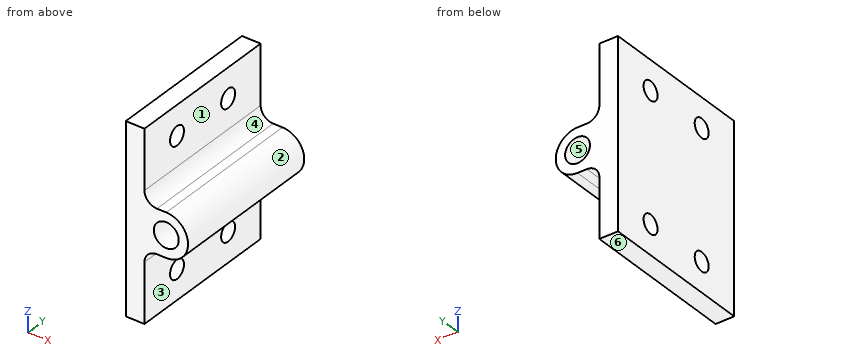
Autodesk Inventor part; units mm, degrees
ref_plane "YZ Plane" through (0, 0, 0) normal (1, 0, 0) x (0, 1, 0)
ref_plane "XZ Plane" through (0, 0, 0) normal (0, 1, 0) x (-1, 0, 0)
ref_plane "XY Plane" through (0, 0, 0) normal (0, 0, 1) x (1, 0, 0)
sketch "Sketch1" plane through (0, 0, 0) normal (0, 1, 0) x (-1, 0, 0)
  line L0 (1.5, 15) -> (-1.5, 15)
  line L1 (-1.5, -15) -> (1.5, -15)
  line L2 (1.5, -15) -> (1.5, 15)
  line L3 (1.5, 15) -> (-1.5, -15) construction
  line L4 (-1.5, 15) -> (1.5, -15) construction
  arc A0 (-5, 3.5) -> (-5, -3.5) centre (-5, 0) ccw
  circle A1 centre (-5, 0) radius 2
  line L5 (-5, -3.5) -> (-3.5, -3.5)
  line L6 (-5, 3.5) -> (-3.5, 3.5)
  line L7 (-1.5, 15) -> (-1.5, 5.5)
  line L8 (-1.5, -5.5) -> (-1.5, -15)
  arc A2 (-3.5, 3.5) -> (-1.5, 5.5) centre (-3.5, 5.5) ccw
  arc A3 (-1.5, -5.5) -> (-3.5, -3.5) centre (-3.5, -5.5) ccw
  point P0 (0, 0)
  dimension "d0" = 3
  dimension "d1" = 30
  dimension "d2" = 7
  dimension "d3" = 4
  dimension "d4" = 2
extrude "Extrusion1" add sketch "Sketch1" along normal blind 25
sketch "Sketch2" plane through (1.5, 0, 15) normal (1, 0, 0) x (0, 0, -1)
  circle A0 centre (4.75, 18) radius 1.5
  circle A1 centre (4.75, 7) radius 1.5
  line L0 (0, 0) -> (0, 25)
  line L1 (0, 25) -> (9.5, 25)
  line L2 (0, 0) -> (9.5, 0)
  point P0 (15, 0)
  dimension "d7" = 3
  dimension "d8" = 3
  dimension "d9" = 4.75
  dimension "d10" = 4.75
  dimension "d11" = 7
  dimension "d15" = 7
extrude "Extrusion2" cut sketch "Sketch2" against normal blind 25
mirror "Mirror1" about plane through (0, 0, 0) normal (0, 0, 1) of "Extrusion2"
properties part number "joint_female"
Input: part model. Units: mm. Frame: model coordinates. Face numbers are marked on the shaded views. A direction names the side the tool comes from. Give positions to 0.01 mm unless a question says otherwise; leave off trailing zeros. Write each loop counter-clockwise with the first axis right and the second up, starting at its lowest first coordinate (ties: lowest second). Pieces come first, ordered by that corner, then holes. Notation, with made-up numbers: (79, -39.75) -> (131, -39.75) arc R14 cw to (131, -21.75) -> close; hole circle Ø8 at (-6, -17.5). An arc over 180 degrees is marked (long way). Use one line per item in the form item = value. Start each with the question number.
1) Section query D-D on z = 10.25. Return the cut outline in (x, y).
2) Draft query along Z for the marked faces 4, 5 and 6. Return one class per face: pulls with the +Z half, pulls with the -Z half, needs draft (parallel to the pull), parting line crosses it, or undercut.
3) Ray query, probe 1 along Y at (x, z) = (0.2, -10.25); probe 2 along X at (y, z) = (23.75, -9.5); probe 3 along Z at (x, y) = (0.5, 6). Return the intervals inside material, ascending. Write a range as from..to.
4) Section query A-A on y = 7. Return the cut outline in (x, z).
5) Set-up query: the marked faces 1, 2 and 3. Return all of +Z, -Z, +X, -X, +Y, -Y with unobstructed straight access to the full face (end or side cutting, diameter ignored); none if empty.
6) Section query C-C on x = 0.5. Return the cut outline in (y, z), then the cut area to 3 significant figures.
7) Pin query (flat end, axial travel): pin 1 (1.6 mm diameter, centred on x = 4.5, y = 18, fed in from +Z); pin 2 (6 mm diameter, centred on x = 2.5, y = 5, fed in from -Z); pin 3 (4 mm diameter, centred on y = 18, z = -10.25, fed in from +X); pin 4 (1.2 mm diameter, centred on x = 4.5, y = 17.5, fed in from -Z). Return the tip coordinate at first contact, or that it passes through.
8) Section query B-B on z = 0. Return the cut outline in (x, y).
Outcome:
q1.outline = (-1.5, 0) -> (1.5, 0) -> (1.5, 5.5) -> (-1.5, 5.5) -> close; (-1.5, 8.5) -> (1.5, 8.5) -> (1.5, 16.5) -> (-1.5, 16.5) -> close; (-1.5, 19.5) -> (1.5, 19.5) -> (1.5, 25) -> (-1.5, 25) -> close
q2.face_4 = pulls with the +Z half
q2.face_5 = undercut
q2.face_6 = pulls with the -Z half
q3.probe_1 = 0..5.5, 8.5..16.5, 19.5..25
q3.probe_2 = -1.5..1.5
q3.probe_3 = -15..-11.37, -9.13..9.13, 11.37..15
q4.outline = (-1.5, -15) -> (1.5, -15) -> (1.5, -11.75) -> (-1.5, -11.75) -> close; (-1.5, -8.75) -> (1.5, -8.75) -> (1.5, -5.5) arc R2 cw to (3.5, -3.5) -> (5, -3.5) arc R3.5 ccw to (5, 3.5) -> (3.5, 3.5) arc R2 cw to (1.5, 5.5) -> (1.5, 8.75) -> (-1.5, 8.75) -> close; (-1.5, 11.75) -> (1.5, 11.75) -> (1.5, 15) -> (-1.5, 15) -> close; hole circle Ø4 at (5, 0)
q5.face_1 = +Z, +X, +Y, -Y
q5.face_2 = +X, +Y, -Y
q5.face_3 = -Z, +X, +Y, -Y
q6.outline = (0, -15) -> (25, -15) -> (25, 15) -> (0, 15) -> close; hole circle Ø3 at (7, -10.25); hole circle Ø3 at (7, 10.25); hole circle Ø3 at (18, -10.25); hole circle Ø3 at (18, 10.25)
q6.area = 722 mm^2
q7.pin_1 = 3.5
q7.pin_2 = -15
q7.pin_3 = 1.5
q7.pin_4 = -3.5
q8.outline = (-1.5, 0) -> (3, 0) -> (3, 25) -> (-1.5, 25) -> close; (7, 0) -> (8.5, 0) -> (8.5, 25) -> (7, 25) -> close
